from build123d import *

# Parameters (mm, degrees)
BODY_BLOCK_DEPTH       = 25
BODY_SHELL_T           = -2
FLOOR_HOLES_DEPTH      = 54.38539126
FLOOR_HOLES_DEPTH_BACK = 54.38539126
SKETCH2_R              = 1.6


with BuildPart() as part:
    # Sketch1 → Body_Block (new body)
    with BuildSketch(Plane.XY):
        with BuildLine():
            Line((-34, -25), (34, -25))
            ThreePointArc((34, -25), (38.242640687, -23.242640687), (40, -19))
            Line((40, -19), (40, 19))
            ThreePointArc((40, 19), (38.242640687, 23.242640687), (34, 25))
            Line((34, 25), (-34, 25))
            ThreePointArc((-34, 25), (-38.242640687, 23.242640687), (-40, 19))
            Line((-40, 19), (-40, -19))
            ThreePointArc((-40, -19), (-38.242640687, -23.242640687), (-34, -25))
        make_face()
    extrude(amount=BODY_BLOCK_DEPTH)

    # Body_Shell
    body_shell_openings = [part.faces().sort_by_distance(p)[0] for p in [
        (0, 0, 25),
    ]]
    offset(amount=BODY_SHELL_T, openings=body_shell_openings, kind=Kind.INTERSECTION)

    # Sketch2 → Floor_Holes (cut, two sides: drawn at the far end of the back side and taken through both)
    with BuildSketch(Plane.XY.offset(-FLOOR_HOLES_DEPTH_BACK)):
        with Locations((-30, -17)):
            Circle(SKETCH2_R)
        with Locations((-30, 17)):
            Circle(SKETCH2_R)
        with Locations((30, -17)):
            Circle(SKETCH2_R)
        with Locations((30, 17)):
            Circle(SKETCH2_R)
    extrude(amount=FLOOR_HOLES_DEPTH + FLOOR_HOLES_DEPTH_BACK, mode=Mode.SUBTRACT)


solid = part.part
Source: CAD feature listing. Evaluate the final solid. Frame: model axes, mm. A direction names the side the tool comes from. Coordinates: 2 decimals unless noted, no trailing zeros. Loops run counter-clockwise (first coordinate to the right, second up) from the corner with the lowest first, then second, coordinate; pieces in that order, holes last. Notation, with made-up numbers: M -22.5,69.25 L 19.5,69.25 A13 cw 19.5,73.25 Z; hole C 73,79.25 d8. An arc over 180 degrees is marked long. Answer in a Markdown table with one row per item.
Q1. Section B-B on y = -17. Return the cut outline in (x, z).
Answers below:
| item | result |
|---|---|
| outline | M -40,0 L -31.6,0 L -31.6,2 L -38,2 L -38,25 L -40,25 Z; M -28.4,0 L 28.4,0 L 28.4,2 L -28.4,2 Z; M 31.6,0 L 40,0 L 40,25 L 38,25 L 38,2 L 31.6,2 Z |
Q2. Draft query along Y for faces 3 (the flat face through (0, 23, 13)), 4 (the cylindrical face through (38.196, -23.289, 12.325)), 5 (the cylindrical face through (38.289, 23.196, 12.325)). Return one class per face: pulls with the +Y half, pulls with the -Y half, needs draft (parallel to the pull), parting line crosses it, or undercut.
Answers below:
| item | result |
|---|---|
| face 3 | undercut |
| face 4 | pulls with the -Y half |
| face 5 | pulls with the +Y half |
Q3. Set-up query: faces 1 (the flat face through (38, 0, 13)), 2 (the flat face through (0, -25, 12)). Return all of +Z, -Z, +X, -X, +Y, -Y with unobstructed straight access to the full face (end or side cutting, diameter ignored); none if empty.
Answers below:
| item | result |
|---|---|
| face 1 | +Z |
| face 2 | +Z, -Z, +X, -X, -Y |
Q4. Section D-D on x = -15.5. Return the cut outline in (y, z), plus the area to 3 significant figures.
Answers below:
| item | result |
|---|---|
| outline | M -25,0 L 25,0 L 25,25 L 23,25 L 23,2 L -23,2 L -23,25 L -25,25 Z |
| area | 192 mm^2 |
Q5. Ray query, probe 1 along X at (y, z) = (17, 1); probe 2 along Y at (x, z) = (30, 1.1); probe 3 along X at (y, z) = (4, 15). Return the intervals inside material, ascending. Write a range as from..to.
Answers below:
| item | result |
|---|---|
| probe 1 | x = -40..-31.6, -28.4..28.4, 31.6..40 |
| probe 2 | y = -25..-18.6, -15.4..15.4, 18.6..25 |
| probe 3 | x = -40..-38, 38..40 |
Q6. First-contact query: pin 1 (3.5 mm diameter, centred on x = -30, y = 17, fed in from +Z). Flat tip, straight axial feed; report the tip coordinate or a pass-through.
Answers below:
| item | result |
|---|---|
| pin 1 | stops at z = 2 |
Q7. Section A-A on x = -30. Return the cut outline in (y, z).
Answers below:
| item | result |
|---|---|
| outline | M -25,0 L -18.6,0 L -18.6,2 L -23,2 L -23,25 L -25,25 Z; M -15.4,0 L 15.4,0 L 15.4,2 L -15.4,2 Z; M 18.6,0 L 25,0 L 25,25 L 23,25 L 23,2 L 18.6,2 Z |
Q8. Section C-C on z = 20.25. Return the cut outline in (x, y), plus the area to 3 significant figures.
Answers below:
| item | result |
|---|---|
| outline | M -40,-19 A6 ccw -34,-25 L 34,-25 A6 ccw 40,-19 L 40,19 A6 ccw 34,25 L -34,25 A6 ccw -40,19 Z; hole M -38,-19 A4 ccw -34,-23 L 34,-23 A4 ccw 38,-19 L 38,19 A4 ccw 34,23 L -34,23 A4 ccw -38,19 Z |
| area | 487 mm^2 |
